CAD build for the part. Positions are in the model's coordinates, mm. Coordinates: 2 decimals unless noted, no trailing zeros. Write each loop counter-clockwise with the first axis right and the second up, starting at its lowest first coordinate (ties: lowest second). Pieces come first, ordered by that corner, then holes. Notation, with made-up numbers: (-6, 9) - (50, 9) arc R24 cw to (50, 22) - close; hole circle Ø9 at (83, 72). An arc over 180 degrees is marked (long way). Answer in a Markdown table with one row per item. Add a question column.
Q1. Band-saw the part on B-B (y = -10.5). List the corners of the cut face in (x, z).
Q2. Band-saw the part on A-A (x = 25). List the corners of the cut face in (y, z).
Q3. Drill centre lines: line 1 along Y through (x, z) = (-25, 1.05); line 2 along Y through (x, z) = (25, 0.85); line 3 along Y through (x, z) = (39, 1.2). Where is each one in solid material? Low to high. Write a range as from..to.
Q4. Pin check, flat tips, straight feed: pin 1 (0.5 mm diameter, centred on x = 43.5, z = 0.5, fed in from -Y); pin 2 (0.5 mm diameter, centred on y = 17.5, z = 0.5, fed in from -X); pin 3 (2 mm diameter, centred on x = 25, y = -15, fed in from -Z); pin 4 (0.8 mm diameter, centred on x = 41, z = 0.5, fed in from -Y). Stop position of each tip, or through.
Q5. Band-saw the part on D-D (z = 0.6). State how many separate pieces and enclosed holes the cut face has, and give its area (3 significant figures).
Q6. Band-saw the part on C-C (x = -25). List the corners of the cut face in (y, z).
Autodesk Fusion 360 part; units mm, degrees
sketch "Sketch1" plane through (0, 0, 0) normal (0, 0, 1) x (1, 0, 0)
  line L0 (45, 27.5) -> (-45, 27.5)
  line L1 (-45, 27.5) -> (-45, -27.5)
  line L2 (-45, -27.5) -> (45, -27.5)
  line L3 (45, -27.5) -> (45, 27.5)
  line L4 (45, 27.5) -> (-45, -27.5) construction
  line L5 (-45, 27.5) -> (45, -27.5) construction
  dimension "d1" = 90
  dimension "d2" = 55
extrude "Extrude1" add sketch "Sketch1" along normal blind 1.6
fillet "Fillet1" radius 5 2 edges at (45, -27.5, 0.8) (45, 27.5, 0.8)
sketch "Sketch2" plane through (0, 0, 1.6) normal (0, 0, 1) x (-1, 0, 0)
  line L0 (45, -27.5) -> (45, 27.5)
  line L1 (45, 27.5) -> (-40, 27.5)
  arc A0 (-40, 27.5) -> (-45, 22.5) centre (-40, 22.5) ccw
  line L2 (-45, 22.5) -> (-45, -22.5)
  arc A1 (-45, -22.5) -> (-40, -27.5) centre (-40, -22.5) ccw
  line L3 (-40, -27.5) -> (45, -27.5)
  line L4 (25, 15) -> (-25, 15) construction
  line L5 (-25, 15) -> (-25, -15)
  line L6 (-25, -15) -> (25, -15) construction
  line L7 (25, -15) -> (25, 15)
  line L8 (25, 15) -> (-25, -15) construction
  line L9 (-25, 15) -> (25, -15) construction
  circle A2 centre (25, -15) radius 2
  circle A3 centre (25, 15) radius 1.8001
  circle A4 centre (-25, 15) radius 1.8646
  circle A5 centre (-25, -15) radius 2
  dimension "d10" = 50
  dimension "d11" = 30
extrude "Extrude2" cut sketch "Sketch2" against normal blind 4 contours A5 | A4 | A3 | A2
sketch "Sketch3" plane through (0, 0, 0) normal (0, 0, -1) x (1, 0, 0)
  circle A0 centre (25, -15) radius 2
  circle A1 centre (25, 15) radius 1.8646
  circle A2 centre (-25, -15) radius 2
  circle A3 centre (-25, 15) radius 1.8001
  line L0 (-45, -27.5) -> (40, -27.5)
  arc A4 (40, -27.5) -> (45, -22.5) centre (40, -22.5) ccw
  line L1 (45, -22.5) -> (45, 22.5)
  arc A5 (45, 22.5) -> (40, 27.5) centre (40, 22.5) ccw
  line L2 (40, 27.5) -> (-45, 27.5)
  line L3 (-45, 27.5) -> (-45, -27.5)
  line L4 (-45, 15) -> (-37, 15)
  line L5 (-37, 15) -> (-37, -15)
  line L6 (-37, -15) -> (-45, -15)
  line L7 (-45, -15) -> (-45, 15)
extrude "Extrude3" cut sketch "Sketch3" against normal blind 3 contours L3 L4 L5 L6 L7
sketch "Sketch4" plane through (0, 0, 0) normal (0, 0, -1) x (1, 0, 0)
  line L0 (-37, -15) -> (-45, -15)
  line L1 (-45, -27.5) -> (40, -27.5)
  arc A0 (40, -27.5) -> (45, -22.5) centre (40, -22.5) ccw
  line L2 (45, -22.5) -> (45, 22.5)
  arc A1 (45, 22.5) -> (40, 27.5) centre (40, 22.5) ccw
  line L3 (40, 27.5) -> (-45, 27.5)
  line L4 (-45, 15) -> (-37, 15)
  line L5 (-37, 15) -> (-37, -15)
  circle A2 centre (25, -15) radius 2
  circle A3 centre (25, 15) radius 1.8646
  circle A4 centre (-25, -15) radius 2
  circle A5 centre (-25, 15) radius 1.8001
  line L6 (45, 15) -> (36, 15)
  line L7 (36, 15) -> (36, -15)
  line L8 (36, -15) -> (45, -15)
  line L9 (45, -15) -> (45, 15)
  line L10 (-45, -15) -> (-45, -27.5)
  line L11 (-45, 27.5) -> (-45, 15)
extrude "Extrude4" cut sketch "Sketch4" against normal blind 6 contours L2 L6 L7 L8 L9
sketch "Sketch5" plane through (0, 0, 1.6) normal (0, 0, 1) x (-1, 0, 0)
  circle A0 centre (25, 15) radius 1.8001
  circle A1 centre (25, -15) radius 2
  circle A2 centre (-25, 15) radius 1.8646
  circle A3 centre (-25, -15) radius 2
  line L0 (45, -15) -> (37, -15)
  line L1 (37, -15) -> (37, 15)
  line L2 (37, 15) -> (45, 15)
  line L3 (45, 27.5) -> (-40, 27.5)
  arc A4 (-40, 27.5) -> (-45, 22.5) centre (-40, 22.5) ccw
  line L4 (-45, -15) -> (-45, -22.5)
  line L5 (-45, 15) -> (-36, 15)
  line L6 (-36, 15) -> (-36, -15)
  line L7 (-36, -15) -> (-45, -15)
  arc A5 (-45, -22.5) -> (-40, -27.5) centre (-40, -22.5) ccw
  line L8 (-40, -27.5) -> (45, -27.5)
  line L9 (-44.8978, -23.5058) -> (-39.8978, -23.5058)
  line L10 (-39.8978, -23.5058) -> (-39.8978, -22.5058)
  line L11 (-39.8978, -22.5058) -> (-45, -22.5)
  line L12 (-45, -21) -> (-40, -21)
  line L13 (-40, -21) -> (-40, -20)
  line L14 (-40, -20) -> (-45, -20)
  line L15 (-45, -18) -> (-40, -18)
  line L16 (-40, -18) -> (-40, -17)
  line L17 (-40, -17) -> (-45, -17)
  line L18 (45, -27.5) -> (45, -15)
  line L19 (45, 15) -> (45, 27.5)
  line L20 (-45, 22.5) -> (-45, 15)
  dimension "d20" = 5
  dimension "d21" = 1
  dimension "d22" = 1
  dimension "d23" = 1
extrude "Extrude5" cut sketch "Sketch5" against normal blind 3 contours A5 L9 L10 L11 | L4 L12 L13 L14 | L4 L15 L16 L17
mirror "Mirror1" about plane through (0, 0, 0) normal (0, 1, 0) of "Extrude5"
sketch "Sketch6" plane through (0, 0, 1.6) normal (0, 0, 1) x (-1, 0, 0)
  circle A0 centre (-25, -15) radius 2
  circle A1 centre (-25, 15) radius 1.8646
  circle A2 centre (25, -15) radius 2
  circle A3 centre (25, 15) radius 1.8001
  line L0 (-44.8978, 23.5058) -> (-39.8978, 23.5058)
  line L1 (-39.8978, 23.5058) -> (-39.8978, 22.5058)
  line L2 (-39.8978, 22.5058) -> (-45, 22.5)
  line L3 (-45, 22.5) -> (-45, 21)
  line L4 (-45, 21) -> (-40, 21)
  line L5 (-40, 21) -> (-40, 20)
  line L6 (-40, 20) -> (-45, 20)
  line L7 (-45, 20) -> (-45, 18)
  line L8 (-45, 18) -> (-40, 18)
  line L9 (-40, 18) -> (-40, 17)
  line L10 (-40, 17) -> (-45, 17)
  line L11 (-45, 15) -> (-36, 15)
  line L12 (-36, 15) -> (-36, -15)
  line L13 (-36, -15) -> (-45, -15)
  line L14 (-45, -17) -> (-40, -17)
  line L15 (-40, -17) -> (-40, -18)
  line L16 (-40, -18) -> (-45, -18)
  line L17 (-45, -18) -> (-45, -20)
  line L18 (-45, -20) -> (-40, -20)
  line L19 (-40, -20) -> (-40, -21)
  line L20 (-40, -21) -> (-45, -21)
  line L21 (-45, -21) -> (-45, -22.5)
  line L22 (-45, -22.5) -> (-39.8978, -22.5058)
  line L23 (-39.8978, -22.5058) -> (-39.8978, -23.5058)
  line L24 (-39.8978, -23.5058) -> (-44.8978, -23.5058)
  arc A4 (-44.8978, -23.5058) -> (-40, -27.5) centre (-40, -22.5) ccw
  line L25 (-40, -27.5) -> (45, -27.5)
  line L26 (45, -15) -> (37, -15)
  line L27 (37, -15) -> (37, 15)
  line L28 (37, 15) -> (45, 15)
  line L29 (45, 27.5) -> (-40, 27.5)
  arc A5 (-40, 27.5) -> (-44.8978, 23.5058) centre (-40, 22.5) ccw
  line L30 (45, -27.5) -> (45, -15)
  line L31 (45, 15) -> (45, 27.5)
  line L32 (-45, 17) -> (-45, 15)
  line L33 (-45, -15) -> (-45, -17)
mirror "Mirror2" about plane through (0, 0, 0) normal (1, 0, 0) of "Extrude5"
mirror "Mirror3" about plane through (0, 0, 0) normal (1, 0, 0) of "Mirror1"
sketch "Sketch7" plane through (-45, 0, 0) normal (-1, 0, 0) x (0, -1, 0)
  line L0 (22.5, 1.6) -> (22.5, 0)
  line L1 (22.5, 0) -> (27.5, 0)
  line L2 (27.5, 0) -> (27.5, 1.6)
  line L3 (27.5, 1.6) -> (22.5, 1.6)
  line L4 (22.5, 1.6) -> (23.5, 1.6)
  line L5 (23.5, 1.6) -> (23.5, 0)
  line L6 (23.5, 0) -> (22.5, 0)
  line L7 (22.5, 0) -> (22.5, 1.6)
extrude "Extrude6" cut sketch "Sketch7" against normal blind 0.5 contours L0 L1 L3 L4 L5 L6 L7
sketch "Sketch8" plane through (-45, 0, 0) normal (-1, 0, 0) x (0, -1, 0)
  line L0 (-22.5, 0) -> (-22.5, 1.6)
  line L1 (-22.5, 1.6) -> (-27.5, 1.6)
  line L2 (-27.5, 1.6) -> (-27.5, 0)
  line L3 (-27.5, 0) -> (-22.5, 0)
  line L4 (-22.5, 1.6) -> (-23.5, 1.6)
  line L5 (-23.5, 1.6) -> (-23.5, 0)
  line L6 (-23.5, 0) -> (-22.5, 0)
  line L7 (-22.5, 0) -> (-22.5, 1.6)
extrude "Extrude7" cut sketch "Sketch8" against normal blind 0.5 contours L0 L1 L3 L4 L5 L6 L7
fillet "Fillet4" radius 2 2 edges at (-45, 27.5, 0.8) (-45, 15, 0.8)
fillet "Fillet5" radius 2 2 edges at (-45, -15, 0.8) (-45, -27.5, 0.8)
fillet "Fillet6" radius 2 4 edges at (45, -15, 0.8) (36, -15, 0.8) (45, 15, 0.8) (36, 15, 0.8)
sketch "Sketch9" plane through (0, 0, 0) normal (0, 0, -1) x (1, 0, 0)
  arc A0 (45, -17) -> (43, -15) centre (43, -17) ccw
  line L0 (43, -15) -> (38, -15)
  arc A1 (36, -13) -> (38, -15) centre (38, -13) ccw
  line L1 (36, -13) -> (36, 13)
  arc A2 (38, 15) -> (36, 13) centre (38, 13) ccw
  line L2 (38, 15) -> (43, 15)
  arc A3 (43, 15) -> (45, 17) centre (43, 17) ccw
  line L3 (45, 17) -> (40, 17)
  line L4 (40, 17) -> (40, 18)
  line L5 (40, 18) -> (45, 18)
  line L6 (45, 18) -> (45, 20)
  line L7 (45, 20) -> (40, 20)
  line L8 (40, 20) -> (40, 21)
  line L9 (40, 21) -> (45, 21)
  line L10 (45, 21) -> (45, 22.5)
  line L11 (45, 22.5) -> (39.8978, 22.5058)
  line L12 (39.8978, 22.5058) -> (39.8978, 23.5058)
  line L13 (39.8978, 23.5058) -> (44.8978, 23.5058)
  arc A4 (44.8978, 23.5058) -> (40, 27.5) centre (40, 22.5) ccw
  line L14 (40, 27.5) -> (-43, 27.5)
  arc A5 (-43, 27.5) -> (-45, 25.5) centre (-43, 25.5) ccw
  line L15 (-45, 25.5) -> (-45, 23.5)
  line L16 (-45, 23.5) -> (-44.899, 23.5)
  arc A6 (-44.8978, 23.5058) -> (-44.899, 23.5) centre (-40, 22.5) ccw
  line L17 (-44.8978, 23.5058) -> (-39.8978, 23.5058)
  line L18 (-39.8978, 23.5058) -> (-39.8978, 22.5058)
  line L19 (-39.8978, 22.5058) -> (-44.5, 22.5006)
  line L20 (-44.5, 22.5006) -> (-44.5, 22.5)
  line L21 (-44.5, 22.5) -> (-45, 22.5)
  line L22 (-45, 22.5) -> (-45, 21)
  line L23 (-45, 21) -> (-40, 21)
  line L24 (-40, 21) -> (-40, 20)
  line L25 (-40, 20) -> (-45, 20)
  line L26 (-45, 20) -> (-45, 18)
  line L27 (-45, 18) -> (-40, 18)
  line L28 (-40, 18) -> (-40, 17)
  line L29 (-40, 17) -> (-45, 17)
  arc A7 (-45, 17) -> (-43, 15) centre (-43, 17) ccw
  line L30 (-43, 15) -> (-37, 15)
  line L31 (-37, 15) -> (-37, -15)
  line L32 (-37, -15) -> (-43, -15)
  arc A8 (-43, -15) -> (-45, -17) centre (-43, -17) ccw
  line L33 (-45, -17) -> (-40, -17)
  line L34 (-40, -17) -> (-40, -18)
  line L35 (-40, -18) -> (-45, -18)
  line L36 (-45, -18) -> (-45, -20)
  line L37 (-45, -20) -> (-40, -20)
  line L38 (-40, -20) -> (-40, -21)
  line L39 (-40, -21) -> (-45, -21)
  line L40 (-45, -21) -> (-45, -22.5)
  line L41 (-45, -22.5) -> (-44.5, -22.5)
  line L42 (-44.5, -22.5) -> (-44.5, -22.5006)
  line L43 (-44.5, -22.5006) -> (-39.8978, -22.5058)
  line L44 (-39.8978, -22.5058) -> (-39.8978, -23.5058)
  line L45 (-39.8978, -23.5058) -> (-44.8978, -23.5058)
  arc A9 (-44.899, -23.5) -> (-44.8978, -23.5058) centre (-40, -22.5) ccw
  line L46 (-44.899, -23.5) -> (-45, -23.5)
  line L47 (-45, -23.5) -> (-45, -25.5)
  arc A10 (-45, -25.5) -> (-43, -27.5) centre (-43, -25.5) ccw
  line L48 (-43, -27.5) -> (40, -27.5)
  arc A11 (40, -27.5) -> (44.8978, -23.5058) centre (40, -22.5) ccw
  line L49 (44.8978, -23.5058) -> (39.8978, -23.5058)
  line L50 (39.8978, -23.5058) -> (39.8978, -22.5058)
  line L51 (39.8978, -22.5058) -> (45, -22.5)
  line L52 (45, -22.5) -> (45, -21)
  line L53 (45, -21) -> (40, -21)
  line L54 (40, -21) -> (40, -20)
  line L55 (40, -20) -> (45, -20)
  line L56 (45, -20) -> (45, -18)
  line L57 (45, -18) -> (40, -18)
  line L58 (40, -18) -> (40, -17)
  line L59 (40, -17) -> (45, -17)
  circle A12 centre (25, -15) radius 2
  circle A13 centre (25, 15) radius 1.8646
  circle A14 centre (-25, -15) radius 2
  circle A15 centre (-25, 15) radius 1.8001
sketch "Sketch10" plane through (0, 0, 1.6) normal (0, 0, 1) x (-1, 0, 0)
  circle A0 centre (25, 15) radius 1.8001
  circle A1 centre (25, -15) radius 2
  circle A2 centre (-25, 15) radius 1.8646
  circle A3 centre (-25, -15) radius 2
  arc A4 (-43, -15) -> (-45, -17) centre (-43, -17) ccw
  line L0 (-45, -17) -> (-40, -17)
  line L1 (-40, -17) -> (-40, -18)
  line L2 (-40, -18) -> (-45, -18)
  line L3 (-45, -18) -> (-45, -20)
  line L4 (-45, -20) -> (-40, -20)
  line L5 (-40, -20) -> (-40, -21)
  line L6 (-40, -21) -> (-45, -21)
  line L7 (-45, -21) -> (-45, -22.5)
  line L8 (-45, -22.5) -> (-39.8978, -22.5058)
  line L9 (-39.8978, -22.5058) -> (-39.8978, -23.5058)
  line L10 (-39.8978, -23.5058) -> (-44.8978, -23.5058)
  arc A5 (-44.8978, -23.5058) -> (-40, -27.5) centre (-40, -22.5) ccw
  line L11 (-40, -27.5) -> (43, -27.5)
  arc A6 (43, -27.5) -> (45, -25.5) centre (43, -25.5) ccw
  line L12 (45, -25.5) -> (45, -23.5)
  line L13 (45, -23.5) -> (44.899, -23.5)
  arc A7 (44.8978, -23.5058) -> (44.899, -23.5) centre (40, -22.5) ccw
  line L14 (44.8978, -23.5058) -> (39.8978, -23.5058)
  line L15 (39.8978, -23.5058) -> (39.8978, -22.5058)
  line L16 (39.8978, -22.5058) -> (44.5, -22.5006)
  line L17 (44.5, -22.5006) -> (44.5, -22.5)
  line L18 (44.5, -22.5) -> (45, -22.5)
  line L19 (45, -22.5) -> (45, -21)
  line L20 (45, -21) -> (40, -21)
  line L21 (40, -21) -> (40, -20)
  line L22 (40, -20) -> (45, -20)
  line L23 (45, -20) -> (45, -18)
  line L24 (45, -18) -> (40, -18)
  line L25 (40, -18) -> (40, -17)
  line L26 (40, -17) -> (45, -17)
  arc A8 (45, -17) -> (43, -15) centre (43, -17) ccw
  line L27 (43, -15) -> (37, -15)
  line L28 (37, -15) -> (37, 15)
  line L29 (37, 15) -> (43, 15)
  arc A9 (43, 15) -> (45, 17) centre (43, 17) ccw
  line L30 (45, 17) -> (40, 17)
  line L31 (40, 17) -> (40, 18)
  line L32 (40, 18) -> (45, 18)
  line L33 (45, 18) -> (45, 20)
  line L34 (45, 20) -> (40, 20)
  line L35 (40, 20) -> (40, 21)
  line L36 (40, 21) -> (45, 21)
  line L37 (45, 21) -> (45, 22.5)
  line L38 (45, 22.5) -> (44.5, 22.5)
  line L39 (44.5, 22.5) -> (44.5, 22.5006)
  line L40 (44.5, 22.5006) -> (39.8978, 22.5058)
  line L41 (39.8978, 22.5058) -> (39.8978, 23.5058)
  line L42 (39.8978, 23.5058) -> (44.8978, 23.5058)
  arc A10 (44.899, 23.5) -> (44.8978, 23.5058) centre (40, 22.5) ccw
  line L43 (44.899, 23.5) -> (45, 23.5)
  line L44 (45, 23.5) -> (45, 25.5)
  arc A11 (45, 25.5) -> (43, 27.5) centre (43, 25.5) ccw
  line L45 (43, 27.5) -> (-40, 27.5)
  arc A12 (-40, 27.5) -> (-44.8978, 23.5058) centre (-40, 22.5) ccw
  line L46 (-44.8978, 23.5058) -> (-39.8978, 23.5058)
  line L47 (-39.8978, 23.5058) -> (-39.8978, 22.5058)
  line L48 (-39.8978, 22.5058) -> (-45, 22.5)
  line L49 (-45, 22.5) -> (-45, 21)
  line L50 (-45, 21) -> (-40, 21)
  line L51 (-40, 21) -> (-40, 20)
  line L52 (-40, 20) -> (-45, 20)
  line L53 (-45, 20) -> (-45, 18)
  line L54 (-45, 18) -> (-40, 18)
  line L55 (-40, 18) -> (-40, 17)
  line L56 (-40, 17) -> (-45, 17)
  arc A13 (-45, 17) -> (-43, 15) centre (-43, 17) ccw
  line L57 (-43, 15) -> (-38, 15)
  arc A14 (-36, 13) -> (-38, 15) centre (-38, 13) ccw
  line L58 (-36, 13) -> (-36, -13)
  arc A15 (-38, -15) -> (-36, -13) centre (-38, -13) ccw
  line L59 (-38, -15) -> (-43, -15)
  line L60 (43, -27.5) -> (-40, -27.5)
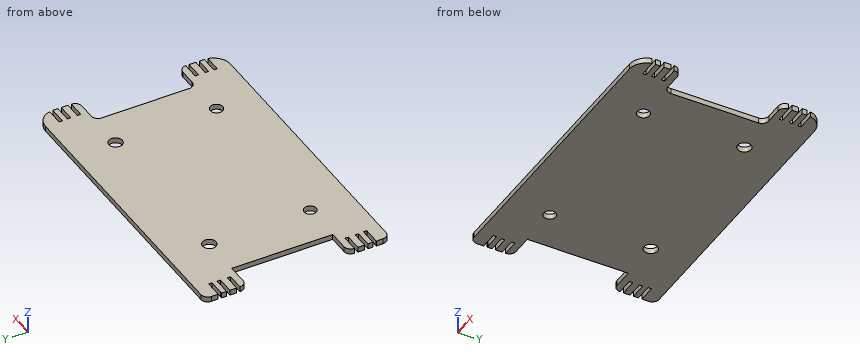
Checked values:
| question | item | result |
|---|---|---|
| 1 | outline | (-37, 0) - (36, 0) - (36, 1.6) - (-37, 1.6) - close |
| 2 | outline | (-27.5, 0) - (-16.86, 0) - (-16.86, 1.6) - (-27.5, 1.6) - close; (-13.14, 0) - (13, 0) - (13, 1.6) - (-13.14, 1.6) - close; (17, 0) - (27.5, 0) - (27.5, 1.6) - (17, 1.6) - close |
| 3 | line 1 | y = -27.5..-16.8, -13.2..13, 17..27.5 |
| 3 | line 2 | y = -27.5..-16.86, -13.14..13, 17..27.5 |
| 3 | line 3 | y = -27.5..-15, 15..27.5 |
| 4 | pin 1 | stops at y = -26.3 |
| 4 | pin 2 | stops at x = -40 |
| 4 | pin 3 | passes through |
| 4 | pin 4 | stops at y = -27.46 |
| 5 | separate pieces | 1 |
| 5 | enclosed holes | 4 |
| 5 | area | 4,320 mm² |
| 6 | outline | (-27.5, 0) - (-16.8, 0) - (-16.8, 1.6) - (-27.5, 1.6) - close; (-13.2, 0) - (13, 0) - (13, 1.6) - (-13.2, 1.6) - close; (17, 0) - (27.5, 0) - (27.5, 1.6) - (17, 1.6) - close |
